```python
from build123d import *

# Parameters (mm, degrees)
SKETCH_W  = 640.1
SKETCH_H  = 19.05
SKETCH_R  = 3
PAD_DEPTH = 19.05


with BuildPart() as part:
    # Sketch → Pad (new body)
    with BuildSketch(Plane.YZ):
        with Locations((320.05, 9.525)):
            Rectangle(SKETCH_W, SKETCH_H)
        with Locations((170.05, 9.525)):
            Circle(SKETCH_R, mode=Mode.SUBTRACT)
        with Locations((470.05, 9.525)):
            Circle(SKETCH_R, mode=Mode.SUBTRACT)
    extrude(amount=PAD_DEPTH)


solid = part.part
```
Verification items for the finished model (mm, model axes). Give positions to 0.01 mm unless a question says otherwise; leave off trailing zeros. One line per item, written item: value.
(1) Scan lines: line 1 along Z through (x, y) = (11.5, 470.05) (3 decimals); line 2 along Y through (x, z) = (2.75, 9); line 3 along Y through (x, z) = (12.75, 8.5). Record each from-to range of solid material in increasing order. Write a range as [from, to].
Final values:
line 1: [0, 6.525], [12.525, 19.05]
line 2: [0, 167.1], [173, 467.1], [473, 640.1]
line 3: [0, 167.23], [172.87, 467.23], [472.87, 640.1]
(2) Gauge pin test, flat end, axial feed: pin 1 (3.5 mm diameter, centred on y = 170.05, z = 9.525, fed in from +X). Record the tip position at first contact, or that the pin passes through.
Final values:
pin 1: through
(3) Draft check along Y on faces 1 (the face through (9, 316, 19.05)), 2 (the face through (9, 640.1, 9)), 3 (the face through (9, 0, 9)). Enter one of: pulls with the +Y half, pulls with the -Y half, needs draft (parallel to the pull), parting line crosses it, or undercut.
Final values:
face 1: needs draft
face 2: pulls with the +Y half
face 3: pulls with the -Y half
